Design review of the part shown in the three views and the two pictorial views. Dimensions are in mm from the part's minimum x, y and z. A direction names the side the tool comes from. Give positions to 0.01 mm unless a question says otherwise; leave off trailing zeros. Order: outer loops, then holes, each group sorted by start corner. A loop starts at its lowest first (then second) coordinate and runs counter-clockwise, first axis right, second up.
Item 1: Consider section C-C (z = 32). Give the boundary of the cut face in (x, y).
Item 2: Consider section B-B (z = 43.5). Give the boundary of the cut face in (x, y), plus the area to 3 significant figures.
Item 3: Consider section A-A (x = 15). Give the boundary of the cut face in (y, z), plus the area to 4 significant figures.
Item 4: For probe 1 along X at (y, z) = (0.65, 43.5); probe 2 along Z at (x, y) = (15, 1.2); probe 3 along Y at (x, z) = (11, 3.5), list the stretches that pass through material, from the lowest coordinate up.
Item 5: Machinability: for the marked faces 1, 2, 3, 4 and 5, which of the approach directions +Z, -Z, +X, -X, +Y, -Y give a long, thin tool a straight path to every point of the face, cutting with its end or side? Answer none if there is none.
Item 6: For P1, Ø8, axis at y = 8, z = 16.5, coming from the -X side; P2, Ø1.5, axis at x = 16, y = 9.5, coming from the -Z side; P3, Ø2.5, axis at x = 15, z = 41.5, coming from the +Y side; P4, Ø15, axis at x = 20.5, z = 14.5, coming from the -Y side, all flat-tipped, find the tip position at first contact; note any pin that passes through.
Item 7: Consider section D-D (x = 6.5). Give the boundary of the cut face in (y, z).
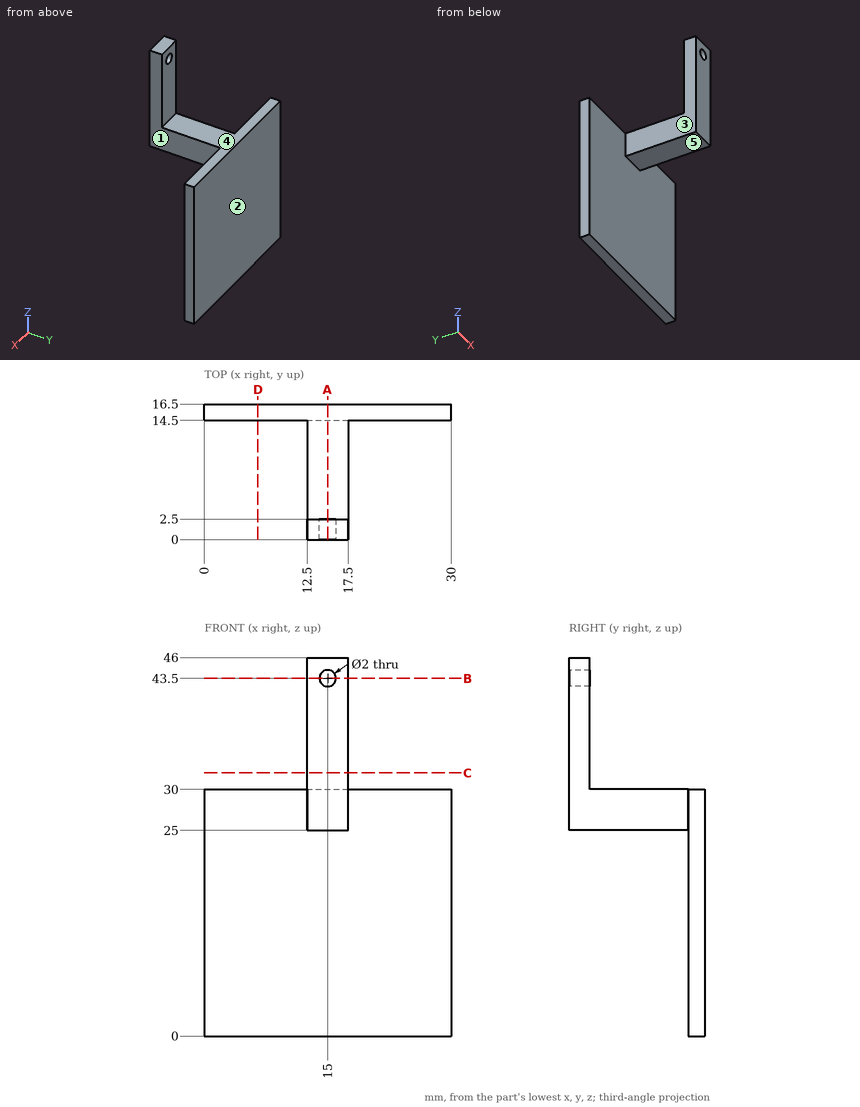
Resolved:
1. outline: (12.5, 0) - (17.5, 0) - (17.5, 2.5) - (12.5, 2.5) - close
2. outline: (12.5, 0) - (14, 0) - (14, 2.5) - (12.5, 2.5) - close; (16, 0) - (17.5, 0) - (17.5, 2.5) - (16, 2.5) - close
2. area: 7.50 mm2
3. outline: (0, 25) - (14.5, 25) - (14.5, 0) - (16.5, 0) - (16.5, 30) - (2.5, 30) - (2.5, 42.5) - (0, 42.5) - close; (0, 44.5) - (2.5, 44.5) - (2.5, 46) - (0, 46) - close
3. area: 167.5 mm2
4. probe 1: x = 12.5 to 14, 16 to 17.5
4. probe 2: z = 25 to 42.5, 44.5 to 46
4. probe 3: y = 14.5 to 16.5
5. face 1: +Z, -Z, +X, -Y
5. face 2: +Z, -Z, +X, -X, +Y
5. face 3: +Z, -Z, -X, -Y
5. face 4: +Z, +X, -X, +Y
5. face 5: -Z, +X, -X, -Y
6. P1: passes through
6. P2: stops at z = 25
6. P3: stops at y = 2.5
6. P4: stops at y = 14.5
7. outline: (14.5, 0) - (16.5, 0) - (16.5, 30) - (14.5, 30) - close
